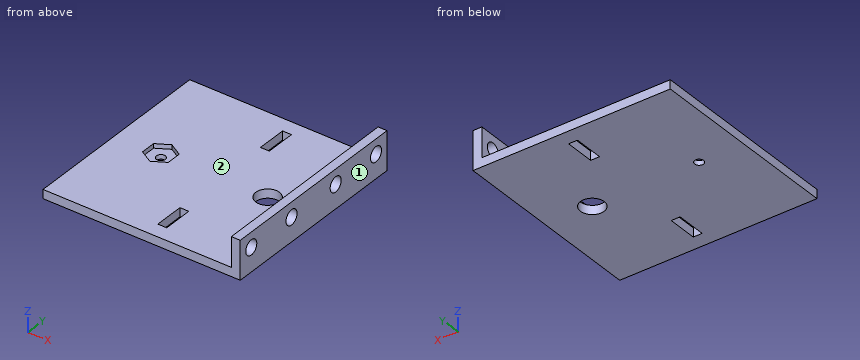
from build123d import *

# Parameters (mm, degrees)
SKETCH1_W           = 66.5
SKETCH1_H           = 66.5
SKETCH1_R           = 4
BOSS_EXTRUDE1_DEPTH = 3
SKETCH3_W           = 3
SKETCH3_H           = 66.5
BOSS_EXTRUDE2_DEPTH = 10
CUT_EXTRUDE1_REACH  = 77.477
SKETCH5_R           = 2.5
CUT_EXTRUDE2_REACH  = 50.787
SKETCH6_W           = 3
SKETCH6_H           = 10
CUT_EXTRUDE5_DEPTH  = 1.5
CUT_EXTRUDE6_REACH  = 50.787
SKETCH9_R           = 1.5


with BuildPart() as part:
    # Sketch1 → Boss-Extrude1 (new body)
    with BuildSketch(Plane.XY):
        Rectangle(SKETCH1_W, SKETCH1_H)
        with Locations((17.75, 0)):
            Circle(SKETCH1_R, mode=Mode.SUBTRACT)
    extrude(amount=BOSS_EXTRUDE1_DEPTH)

    # Sketch3 → Boss-Extrude2 (add)
    with BuildSketch(Plane.XY.offset(3)):
        with Locations((31.75, 0)):
            Rectangle(SKETCH3_W, SKETCH3_H)
    extrude(amount=BOSS_EXTRUDE2_DEPTH)

    # Sketch5 → Cut-Extrude1 (cut, up to next)
    with BuildSketch(Plane(origin=(33.25, 0, 0), x_dir=(0, 0, -1), z_dir=(1, 0, 0)), mode=Mode.PRIVATE) as cut_extrude1_sk1:
        with Locations(Location((-8, -28.25, 0), (0, 0, 90))):
            Circle(SKETCH5_R)
    cut_extrude1_tool1 = extrude(cut_extrude1_sk1.sketch, amount=-CUT_EXTRUDE1_REACH, mode=Mode.PRIVATE) & part.part
    # Sketch5 → Cut-Extrude1 (cut, up to next)
    with BuildSketch(Plane(origin=(33.25, 0, 0), x_dir=(0, 0, -1), z_dir=(1, 0, 0)), mode=Mode.PRIVATE) as cut_extrude1_sk2:
        with Locations(Location((-8, -10, 0), (0, 0, 90))):
            Circle(SKETCH5_R)
    cut_extrude1_tool2 = extrude(cut_extrude1_sk2.sketch, amount=-CUT_EXTRUDE1_REACH, mode=Mode.PRIVATE) & part.part
    cut_extrude1_1 = cut_extrude1_tool1.solids().sort_by_distance((33.25, -28.25, 8))[0]
    add(cut_extrude1_1, mode=Mode.SUBTRACT)
    cut_extrude1_2 = cut_extrude1_tool2.solids().sort_by_distance((33.25, -10, 8))[0]
    add(cut_extrude1_2, mode=Mode.SUBTRACT)
    cut_extrude1 = cut_extrude1_1 + cut_extrude1_2  # Cut-Extrude1 as one shape, for the pattern or mirror that repeats it

    # Mirror2: Cut-Extrude1 across plane
    add(cut_extrude1.mirror(Plane.ZX), mode=Mode.SUBTRACT)

    # Sketch6 → Cut-Extrude2 (cut, up to next)
    with BuildSketch(Plane(origin=(0, 0, 0), x_dir=(-1, 0, 0), z_dir=(0, 0, -1)), mode=Mode.PRIVATE) as cut_extrude2_sk1:
        with Locations((-3.25, 23.25)):
            Rectangle(SKETCH6_W, SKETCH6_H)
    cut_extrude2_tool1 = extrude(cut_extrude2_sk1.sketch, amount=-CUT_EXTRUDE2_REACH, mode=Mode.PRIVATE) & part.part
    cut_extrude2 = cut_extrude2_tool1.solids().sort_by_distance((3.25, 23.25, 0))[0]
    add(cut_extrude2, mode=Mode.SUBTRACT)

    # Mirror3: Cut-Extrude2 across plane
    add(cut_extrude2.mirror(Plane.ZX), mode=Mode.SUBTRACT)

    # Sketch7 → Cut-Extrude5 (cut)
    with BuildSketch(Plane(origin=(0, 0, 3), x_dir=(-1, 0, 0), z_dir=(0, 0, -1))):
        Polygon((18.25, -5), (22.580127019, -2.5), (22.580127019, 2.5), (18.25, 5), (13.919872981, 2.5), (13.919872981, -2.5), align=None)
    extrude(amount=CUT_EXTRUDE5_DEPTH, mode=Mode.SUBTRACT)

    # Sketch9 → Cut-Extrude6 (cut, up to next)
    with BuildSketch(Plane(origin=(0, 0, 0), x_dir=(-1, 0, 0), z_dir=(0, 0, -1)), mode=Mode.PRIVATE) as cut_extrude6_sk1:
        with Locations((18.25, 0)):
            Circle(SKETCH9_R)
    cut_extrude6_tool1 = extrude(cut_extrude6_sk1.sketch, amount=-CUT_EXTRUDE6_REACH, mode=Mode.PRIVATE) & part.part
    add(cut_extrude6_tool1.solids().sort_by_distance((-18.25, 0, 0))[0], mode=Mode.SUBTRACT)


solid = part.part
Design review of the part built by this model. Coordinates are the model's own, in mm. Face numbers are marked on the shaded views. A direction names the side the tool comes from. Round coordinates to 2 decimals unless told otherwise and drop trailing zeros. Order: outer loops, then holes, each group sorted by start corner. A loop starts at its lowest first (then second) coordinate and runs counter-clockwise, first axis right, second up. Notation, with made-up numbers: M 53.5,9 L 107.5,9 A19 cw 107.5,20 Z; hole C 23.25,-1 d7. An arc over 180 degrees is marked long. Answer as CSV lines item,"result". Start each with the question number.
1) Add section D-D (y = 0). Give the boundary of the cut face in (x, z).
2) For pin 1 Ø9.5 at (x, y) = (-17, 1.5) entering from +Z, flat-tipped, find the tip position at first contact; note if it passes through.
3) Tool access review of the marked faces 1 and 2: name each direction out of +Z, -Z, +X, -X, +Y, -Y from which nothing blocks a thin tool from reaching the whole face with its end or side.
4) Add section A-A (y = -21.5). Give the boundary of the cut face in (x, z).
5) Wall thickness on line 1 along Y through (x, z) = (-18.25, 1.1); line 2 along Z through (x, y) = (30.95, -28.25); line 3 along X through (y, z) = (1.5, 2.75): over which ranges is each line inside the solid? List them lowest first. Write a range as [from, to].
6) Add section C-C (z = 6.5). Give the boundary of the cut face in (x, y), then the cut area to 4 significant figures.
7) Add section B-B (x = 17.75). Give the boundary of the cut face in (y, z), then the cut area to 4 significant figures.
Resolved:
1,outline,"M -33.25,0 L -19.75,0 L -19.75,1.5 L -22.58,1.5 L -22.58,3 L -33.25,3 Z; M -16.75,0 L 13.75,0 L 13.75,3 L -13.92,3 L -13.92,1.5 L -16.75,1.5 Z; M 21.75,0 L 33.25,0 L 33.25,13 L 30.25,13 L 30.25,3 L 21.75,3 Z"
2,pin 1,"z = 3"
3,face 1,"+Z, -Z, +X, +Y, -Y"
3,face 2,"+Z, -X, +Y, -Y"
4,outline,"M -33.25,0 L 1.75,0 L 1.75,3 L -33.25,3 Z; M 4.75,0 L 33.25,0 L 33.25,13 L 30.25,13 L 30.25,3 L 4.75,3 Z"
5,line 1,"[-33.25, -1.5], [1.5, 33.25]"
5,line 2,"[0, 5.5], [10.5, 13]"
5,line 3,"[-33.25, -22.58], [-13.92, 14.04], [21.46, 33.25]"
6,outline,"M 30.25,-33.25 L 33.25,-33.25 L 33.25,-30.25 L 30.25,-30.25 Z; M 30.25,-26.25 L 33.25,-26.25 L 33.25,-12 L 30.25,-12 Z; M 30.25,-8 L 33.25,-8 L 33.25,8 L 30.25,8 Z; M 30.25,12 L 33.25,12 L 33.25,26.25 L 30.25,26.25 Z; M 30.25,30.25 L 33.25,30.25 L 33.25,33.25 L 30.25,33.25 Z"
6,area,"151.5 mm^2"
7,outline,"M -33.25,0 L -4,0 L -4,3 L -33.25,3 Z; M 4,0 L 33.25,0 L 33.25,3 L 4,3 Z"
7,area,"175.5 mm^2"
